CAD build for the part. Positions are in the model's coordinates, mm. A direction names the side the tool comes from. Coordinates: 2 decimals unless noted, no trailing zeros. Loops run counter-clockwise (first coordinate to the right, second up) from the corner with the lowest first, then second, coordinate; pieces in that order, holes last. Notation, with made-up numbers: (-27.5, 66) -> (0.5, 66) arc R19 ccw to (0.5, 84) -> close; hole circle Ø2 at (31, -18.75). An arc over 180 degrees is marked (long way). Answer as CSV lines item,"result". Start each with the question number.
from build123d import *

# Parameters (mm, degrees)
SKETCH_W      = 36.48
SKETCH_H      = 12
PAD_DEPTH     = 1.5
PAD001_DEPTH  = 2.5
SKETCH002_W   = 3.6
SKETCH002_H   = 1.5
SKETCH002_W_2 = 1.5
SKETCH002_H_2 = 3.6
PAD002_DEPTH  = 4
FILLET_R      = 1


with BuildPart() as part:
    # Sketch → Pad (new body)
    with BuildSketch(Plane.XY):
        with Locations((-18.24, 0)):
            Rectangle(SKETCH_W, SKETCH_H)
    pad = extrude(amount=PAD_DEPTH)

    # Sketch001 → Pad001 (join)
    with BuildSketch(Plane.XY.offset(1.5)):
        Polygon((-36.48, 6), (0, 6), (0, 4.5), (-34.98, 4.5), (-34.98, -4.5), (0, -4.5), (0, -6), (-36.48, -6), align=None)
    pad001 = extrude(amount=PAD001_DEPTH)

    # Sketch002 → Pad002 (join)
    with BuildSketch(Plane.XY):
        with Locations((-30.48, 2.65)):
            Rectangle(SKETCH002_W, SKETCH002_H)
        with Locations((-30.48, -2.65)):
            Rectangle(SKETCH002_W, SKETCH002_H)
        with Locations((-33.13, 0)):
            Rectangle(SKETCH002_W_2, SKETCH002_H_2)
        with Locations((-27.83, 0)):
            Rectangle(SKETCH002_W_2, SKETCH002_H_2)
    pad002 = extrude(amount=PAD002_DEPTH)

    # Mirrored: Pad across Sketch V_Axis
    add(pad.mirror(Plane(origin=(0, 0, 0), x_dir=(0, 0, 1), z_dir=(1, 0, 0))))

    # Mirrored001: Pad002 across Sketch002 V_Axis
    add(pad002.mirror(Plane(origin=(0, 0, 0), x_dir=(0, 0, 1), z_dir=(1, 0, 0))))

    # Mirrored002: Pad001 across Sketch001 V_Axis
    add(pad001.mirror(Plane(origin=(0, 0, 1.5), x_dir=(0, 0, 1), z_dir=(1, 0, 0))))

    # Fillet
    fillet_edges = [part.edges().sort_by_distance(p)[0] for p in [
        (36.48, 0, 0),
        (0, -6, 0),
        (-36.48, 0, 0),
        (0, 6, 0),
    ]]
    fillet(fillet_edges, radius=FILLET_R)


solid = part.part
Item 1: Wall check: probe 1 along X at (y, z) = (-0.75, 2.15); probe 2 along X at (y, z) = (-3, 2.9); probe 3 along Y at (x, z) = (-23, 2.85). Give the ranges that are in metal, low to high.
Item 2: Which spindle directions (+Z, -Z, +X, -X, +Y, -Y) get a long thin tool onto all of the face, cutting with end or side? Do faces 1 (the face through (-32.28, -3, 3)), 2 (the face through (-28, 0, 4)). Say none if no direction does.
Item 3: Saw through at A-A (z = 2.7). Count the separate pieces of the cut face and the enclosed holes in it, plus the area to 3 significant figures.
Item 4: Saw through at B-B (x = -11.5). Write the cut outline in (y, z).
Item 5: Flat gauge pin, fed straight in: pin 1 Ø1.5 at (x, y) = (13, 4) entering from +Z. Where does the tip first touch, or does it go through?
Item 6: Two-plate mould, pull along X, no slides. Class faces 3 (the face through (0, -4.5, 3)), 4 (the face through (-1, -6, 2)), 5 (the face through (36.48, 0, 2)): pulls with the +X half, pulls with the -X half, needs draft (parallel to the pull), parting line crosses it, or undercut.
Item 7: Saw through at C-C (y = -0.25). Write the cut outline in (x, z).
Geometry check:
1,probe 1,"-36.48 to -34.98, -33.88 to -32.38, -28.58 to -27.08, 27.08 to 28.58, 32.38 to 33.88, 34.98 to 36.48"
1,probe 2,"-36.48 to -34.98, -32.28 to -28.68, 28.68 to 32.28, 34.98 to 36.48"
1,probe 3,"-6 to -4.5, 4.5 to 6"
2,face 1,"+Z"
2,face 2,"+Z, +X, -X, +Y, -Y"
3,separate pieces,"9"
3,enclosed holes,"1"
3,area,"289 mm2"
4,outline,"(-6, 1) arc R1 ccw to (-5, 0) -> (5, 0) arc R1 ccw to (6, 1) -> (6, 4) -> (4.5, 4) -> (4.5, 1.5) -> (-4.5, 1.5) -> (-4.5, 4) -> (-6, 4) -> close"
5,pin 1,"z = 4"
6,face 3,"undercut"
6,face 4,"needs draft"
6,face 5,"pulls with the +X half"
7,outline,"(-36.48, 1) arc R1 ccw to (-35.48, 0) -> (35.48, 0) arc R1 ccw to (36.48, 1) -> (36.48, 4) -> (34.98, 4) -> (34.98, 1.5) -> (33.88, 1.5) -> (33.88, 4) -> (32.38, 4) -> (32.38, 1.5) -> (28.58, 1.5) -> (28.58, 4) -> (27.08, 4) -> (27.08, 1.5) -> (-27.08, 1.5) -> (-27.08, 4) -> (-28.58, 4) -> (-28.58, 1.5) -> (-32.38, 1.5) -> (-32.38, 4) -> (-33.88, 4) -> (-33.88, 1.5) -> (-34.98, 1.5) -> (-34.98, 4) -> (-36.48, 4) -> close"
